Source: CAD feature listing. Evaluate the final solid. Frame: model axes, mm. A direction names the side the tool comes from. Give positions to 0.01 mm unless a question says otherwise; leave off trailing zeros. Order: outer loops, then holes, each group sorted by start corner. A loop starts at its lowest first (then second) coordinate and runs counter-clockwise, first axis right, second up. Notation, with made-up numbers: M 88,59.25 L 143,59.25 A30 cw 143,87.25 Z; hole C 1,57.25 d4. An arc over 180 degrees is marked long. Answer in a Markdown table with one row per item. Add a question column.
(1) Section query B-B, the plane x = 0. Return loops of the section in (y, z), plus the area to 3 significant figures.
(2) Set-up query: faces 1 (the face through (-4.276, 16.757, 0.39)), 2 (the face through (-0.541, 3.283, -4.276)), 3 (the face through (1.83, 9.86, 5.82)). Return all of +Z, -Z, +X, -X, +Y, -Y with unobstructed straight access to the full face (end or side cutting, diameter ignored); none if empty.
(3) Pin query (flat end, axial travel): P1, Ø2, axis at y = 6, z = -3, coming from the -X side; P2, Ø2, axis at y = 5, z = 0, coming from the -X side; P3, Ø3, axis at y = 12, z = -4, coming from the -X side. Return the tip coordinate at first contact, or that it passes through.
(4) Material intervals for line 1 along Y through (x, z) = (0, -3.2); line 2 along X through (y, z) = (13, 0); line 3 along Y through (x, z) = (-4, 1.5), sorted ascending.
(5) Section query A-A, the plane z = 0. Return loops of the section in (x, y), plus the area to 3 significant figures.
(6) Section query C-C, the plane y = 16.25. Return loops of the section in (x, z), plus the area to 3 significant figures.
(7) Section query D-D, the plane z = 2.5. Return loops of the section in (x, y), plus the area to 3 significant figures.
(8) Mould query, pull axis Y, two halves, no side actions, for faces 4 (the face through (3, 20, 1)), 5 (the face through (-4.276, 3.215, 0.234)), 6 (the face through (3, 0, 1)). Classes: pulls with the +Y half, pulls with the -Y half, needs draft (parallel to the pull), parting line crosses it, or undercut.
from build123d import *

# Parameters (mm, degrees)
CROQUIS1_R                            = 6.1
SALIENTE_EXTRUIR1_DEPTH               = 20
CROQUIS3_R                            = 3
CORTAR_EXTRUIR1_DEPTH                 = 22.781184541
CROQUIS5_W                            = 1.8
CROQUIS5_H                            = 6.1
TALADRO_DE_MARGEN_PARA_M31_AT_2_COUNT = 2
TALADRO_DE_MARGEN_PARA_M31_AT_2_PITCH = 10
CROQUIS7_W                            = 1.8
CROQUIS7_H                            = 6.1
TALADRO_DE_MARGEN_PARA_M32_AT_2_COUNT = 2
TALADRO_DE_MARGEN_PARA_M32_AT_2_PITCH = 10


with BuildPart() as part:
    # Croquis1 → Saliente-Extruir1 (new body)
    with BuildSketch(Plane(origin=(0, 0, 0), x_dir=(-1, 0, 0), z_dir=(0, 1, 0))):
        with Locations(Location((0, 0, 0), (0, 0, 90))):
            Circle(CROQUIS1_R)
    extrude(amount=SALIENTE_EXTRUIR1_DEPTH)

    # Croquis3 → Cortar-Extruir1 (cut, through all)
    with BuildSketch(Plane.XZ):
        with Locations(Location((0, 0, 0), (0, 0, 270))):
            Circle(CROQUIS3_R)
    extrude(amount=-CORTAR_EXTRUIR1_DEPTH, mode=Mode.SUBTRACT)

    # Croquis5 → Taladro de margen para M31 (revolve, cut)
    with BuildSketch(Plane(origin=(0, 15, 0), x_dir=(0, -1, 0), z_dir=(1, 0, 0))):
        with Locations((0.9, 3.05)):
            Rectangle(CROQUIS5_W, CROQUIS5_H)
    taladro_de_margen_para_m31 = revolve(axis=Axis((0, 15, 6.35), (0, 0, -1)), mode=Mode.SUBTRACT)

    # Taladro de margen para M31 at 2: Taladro de margen para M31 ×2
    with Locations(*[(0, -i * TALADRO_DE_MARGEN_PARA_M31_AT_2_PITCH, 0) for i in range(1, TALADRO_DE_MARGEN_PARA_M31_AT_2_COUNT)]):
        add(taladro_de_margen_para_m31, mode=Mode.SUBTRACT)

    # Croquis7 → Taladro de margen para M32 (revolve, cut)
    with BuildSketch(Plane(origin=(0, 5, 0), x_dir=(0, 0, -1), z_dir=(0, 1, 0))):
        with Locations((0.9, 3.05)):
            Rectangle(CROQUIS7_W, CROQUIS7_H)
    taladro_de_margen_para_m32 = revolve(axis=Axis((6.35, 5, 0), (-1, 0, 0)), mode=Mode.SUBTRACT)

    # Taladro de margen para M32 at 2: Taladro de margen para M32 ×2
    with Locations(*[(0, i * TALADRO_DE_MARGEN_PARA_M32_AT_2_PITCH, 0) for i in range(1, TALADRO_DE_MARGEN_PARA_M32_AT_2_COUNT)]):
        add(taladro_de_margen_para_m32, mode=Mode.SUBTRACT)


solid = part.part
Values follow:
| question | item | result |
|---|---|---|
| 1 | outline | M 0,-6.1 L 3.2,-6.1 L 3.2,-3 L 0,-3 Z; M 0,3 L 20,3 L 20,6.1 L 0,6.1 Z; M 6.8,-6.1 L 13.2,-6.1 L 13.2,-3 L 6.8,-3 Z; M 16.8,-6.1 L 20,-6.1 L 20,-3 L 16.8,-3 Z |
| 1 | area | 102 mm² |
| 2 | face 1 | -X |
| 2 | face 2 | -Z |
| 2 | face 3 | +Y, -Y |
| 3 | P1 | stops at x = -5.76 |
| 3 | P2 | stops at x = 2.83 |
| 3 | P3 | stops at x = -5.56 |
| 4 | line 1 | y = 0 to 3.2, 6.8 to 13.2, 16.8 to 20 |
| 4 | line 2 | x = -6.1 to -3, 3 to 6.1 |
| 4 | line 3 | y = 0 to 4.01, 5.99 to 14.01, 15.99 to 20 |
| 5 | outline | M -6.1,0 L -3,0 L -3,3.2 L -6.1,3.2 Z; M -6.1,6.8 L -3,6.8 L -3,13.2 L -6.1,13.2 Z; M -6.1,16.8 L -3,16.8 L -3,20 L -6.1,20 Z; M 3,0 L 6.1,0 L 6.1,20 L 3,20 Z |
| 5 | area | 102 mm² |
| 6 | outline | M -5.96,-1.3 A6.1 ccw -1.3,-5.96 L -1.3,-2.71 A3 cw -2.71,-1.3 Z; M -5.96,1.3 L -2.71,1.3 A3 cw long 1.3,-2.71 L 1.3,-5.96 A6.1 ccw long Z |
| 6 | area | 72.3 mm² |
| 7 | outline | M -5.56,0 L -1.66,0 L -1.66,20 L -5.56,20 Z; M 1.66,0 L 5.56,0 L 5.56,20 L 1.66,20 Z |
| 7 | area | 156 mm² |
| 8 | face 4 | pulls with the +Y half |
| 8 | face 5 | undercut |
| 8 | face 6 | pulls with the -Y half |
